Solid Edge part; units mm, degrees
sketch "Sketch1" plane through (0, 0, 0) normal (0, -1, 0) x (1, 0, 0)
  line L0 (0, 0) -> (-49.3, 0)
  line L1 (-49.3, 0) -> (-49.3, 50)
  line L2 (-49.3, 50) -> (-20.7107, 50)
  line L3 (-20.7107, 50) -> (0, 0)
  dimension "D1" = 49.3
extrude "Protrusion1" add sketch "Sketch1" against normal blind 50
hole "Bohrung_1" at (-49.3, 36, 32.5) direction (1, 0, 0) diameter 4.917 depth 24 tip angle 118 thread major 6 thread length 18
hole "Hole1" at (-49.3, 10, 14.5) direction (1, 0, 0) diameter 4.917 depth 24 tip angle 118 thread major 6 thread length 18
hole "Bohrung_3" at (-33.3, 21.5, 0) direction (0, 0, 1) diameter 3.242 depth 16 tip angle 118 thread major 4 thread length 12
properties part number "A1.2-A" material "AlMgSi 0,5-1"
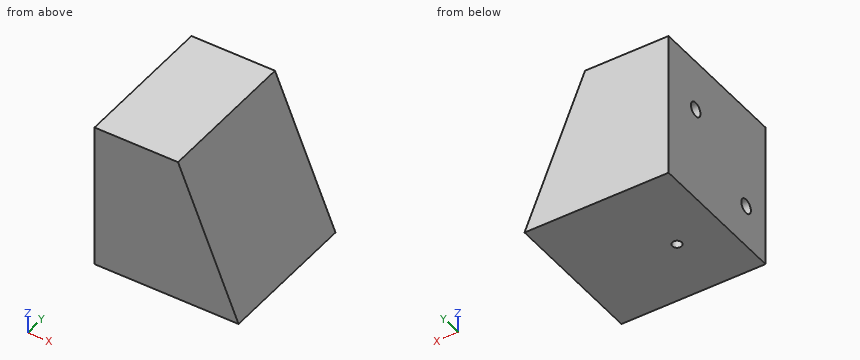
Check sheet for the modelled part. Datum: model origin and axes. Units: mm. Give positions to 0.01 mm unless a question says otherwise; leave off trailing zeros. Write each loop counter-clockwise with the first axis right and the second up, starting at its lowest first coordinate (ties: lowest second). Pieces come first, ordered by that corner, then holes. Notation, with made-up numbers: M 65,87 L 115,87 A7 cw 115,100 Z; hole C 89,66.25 d7. An arc over 180 degrees is marked long. Use one line per item in the form item = value.
(1) Material ranges on line 1 along Z through (x, y) = (-37, 10); line 2 along Y through (x, z) = (-33.3, 8.5); line 3 along Y through (x, z) = (-40.5, 32.5), recorded low to high.
Answer block:
line_1 = 0 to 12.04, 16.96 to 50
line_2 = 0 to 19.88, 23.12 to 50
line_3 = 0 to 33.54, 38.46 to 50
(2) Section check C-C on y = 13.5. Record the boundary of the cut face in (x, z).
Answer block:
outline = M -49.3,0 L 0,0 L -20.71,50 L -49.3,50 Z
(3) Section check A-A on x = -29.5. Record the boundary of the cut face in (y, z), plus the area to 3 significant figures.
Answer block:
outline = M 0,0 L 50,0 L 50,50 L 0,50 Z; hole C 10,14.5 d4.92; hole C 36,32.5 d4.92
area = 2,460 mm2
(4) Section check D-D on x = -13.5. Record the boundary of the cut face in (y, z).
Answer block:
outline = M 0,0 L 50,0 L 50,32.59 L 0,32.59 Z
(5) Section check B-B on z = 10.5. Record the boundary of the cut face in (x, y).
Answer block:
outline = M -49.3,0 L -4.35,0 L -4.35,50 L -49.3,50 Z; hole C -33.3,21.5 d3.24
(6) Depth check by flat-ended pin: P1, Ø1.9, axis at x = -33.3, y = 21.5, coming from the -Z side; P2, Ø6, axis at x = -19.5, y = 23, coming from the -Z side; P3, Ø3, axis at y = 10, z = 14.5, coming from the +X side; P4, Ø1.5, axis at y = 36.5, z = 17, coming from the +X side. Enter the tip coordinate at first touch or a pass-through.
Answer block:
P1 = 16.4
P2 = 0
P3 = -5.38
P4 = -6.73
